from build123d import *

# Parameters (mm, degrees)
CROQUIS1_R              = 1.5875
SALIENTE_EXTRUIR1_DEPTH = 10.4775
CROQUIS2_R              = 3.175
SALIENTE_EXTRUIR2_DEPTH = 3.175
CORTAR_EXTRUIR5_DEPTH   = 2.794


with BuildPart() as part:
    # Croquis1 → Saliente-Extruir1 (new body)
    with BuildSketch(Plane.XY):
        Circle(CROQUIS1_R)
    extrude(amount=-SALIENTE_EXTRUIR1_DEPTH)

    # Croquis2 → Saliente-Extruir2 (add)
    with BuildSketch(Plane.XY):
        Circle(CROQUIS2_R)
    extrude(amount=SALIENTE_EXTRUIR2_DEPTH)

    # Croquis3 → Cortar-Extruir5 (cut)
    with BuildSketch(Plane.XY.offset(3.175)):
        Polygon((2.294680271, -1.089055764), (2.090490093, 1.442723526), (-0.204190178, 2.53177929), (-2.294680271, 1.089055764), (-2.090490093, -1.442723526), (0.204190178, -2.53177929), align=None)
    extrude(amount=-CORTAR_EXTRUIR5_DEPTH, mode=Mode.SUBTRACT)


solid = part.part
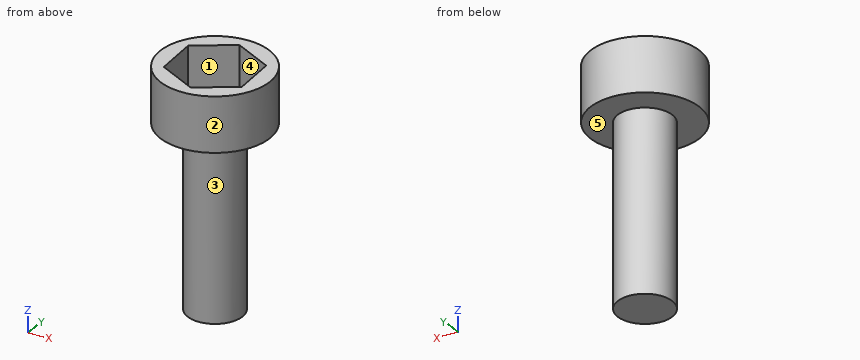
The model under review builds one solid part; all positions refer to its coordinate system, in mm. Face numbers are marked on the shaded views. A direction names the side the tool comes from. Coordinates: 2 decimals unless noted, no trailing zeros. Loops run counter-clockwise (first coordinate to the right, second up) from the corner with the lowest first, then second, coordinate; pieces in that order, holes last.
(1) Insertion check: P1, Ø3, axis at x = 2, z = -4, coming from the +Y side; P2, Ø3, axis at y = 2.5, z = 0.5, coming from the -X side; P3, Ø1.4, axis at x = 1, y = 0, coming from the +Z side. Each pin has a flat end and moves straight along its axis. Give the tip position at first contact, or say it passes through.
Determined:
P1: stops at y = 1.51
P2: stops at x = -3.01
P3: stops at z = 0.38
(2) Consider section B-B, the plane z = -5.25. Give the boundary of the cut face in (x, y) (1 decimal).
Determined:
outline: circle Ø3.2 at (0, 0)
(3) Draft analysis for pull direction X (two halves, no side actions). For the marked faces 3, 4 and 5, state which applies: +X half, -X half, draft (parallel to the pull), parting line (faces both ways), or undercut.
Determined:
face 3: parting line
face 4: undercut
face 5: draft
(4) Consider section A-A, the plane y = -2. Give the boundary of the cut face in (x, z) (3 decimals).
Determined:
outline: (-2.466, 0) - (2.466, 0) - (2.466, 3.175) - (0.975, 3.175) - (0.975, 0.381) - (-0.916, 0.381) - (-0.916, 3.175) - (-2.466, 3.175) - close
(5) Wall thickness on L1, parallel to Y at x = 0, z = -4.25; L2, parallel to Y at x = -1, z = 2.5; L3, parallel to Z at x = 0.5, y = 1.25: over which ranges is each line inside the solid? List them lowest first.
Determined:
L1: y = -1.59 to 1.59
L2: y = -3.01 to -1.96, 1.98 to 3.01
L3: z = -10.48 to 0.38
(6) Tool access review of the marked faces 1 and 2: name each direction out of +Z, -Z, +X, -X, +Y, -Y from which nothing blocks a thin tool from reaching the whole face with its end or side.
Determined:
face 1: +Z
face 2: +Z, -Z
(7) Consider section D-D, the plane y = -0.5. Give the boundary of the cut face in (x, z) (1 decimal).
Determined:
outline: (-3.1, 0) - (-1.5, 0) - (-1.5, -10.5) - (1.5, -10.5) - (1.5, 0) - (3.1, 0) - (3.1, 3.2) - (2.2, 3.2) - (2.2, 0.4) - (-2.2, 0.4) - (-2.2, 3.2) - (-3.1, 3.2) - close
(8) Consider section C-C, the plane x = 0. Give the boundary of the cut face in (y, z) (1 decimal).
Determined:
outline: (-3.2, 0) - (-1.6, 0) - (-1.6, -10.5) - (1.6, -10.5) - (1.6, 0) - (3.2, 0) - (3.2, 3.2) - (2.4, 3.2) - (2.4, 0.4) - (-2.4, 0.4) - (-2.4, 3.2) - (-3.2, 3.2) - close
